Geometry check sheet. Reference: drawing and pictorial views, mm from the part's lowest x, y, z. Coordinates: 2 decimals unless noted, no trailing zeros. Write each loop counter-clockwise with the first axis right and the second up, starting at its lowest first coordinate (ties: lowest second). Pieces come first, ordered by that corner, then holes. Notation, with made-up numbers: (16.25, 57) -> (39.25, 57) arc R15 ccw to (39.25, 69) -> close; hole circle Ø4 at (-21.5, 45). An arc over 180 degrees is marked (long way). Use a Markdown table: item, result.
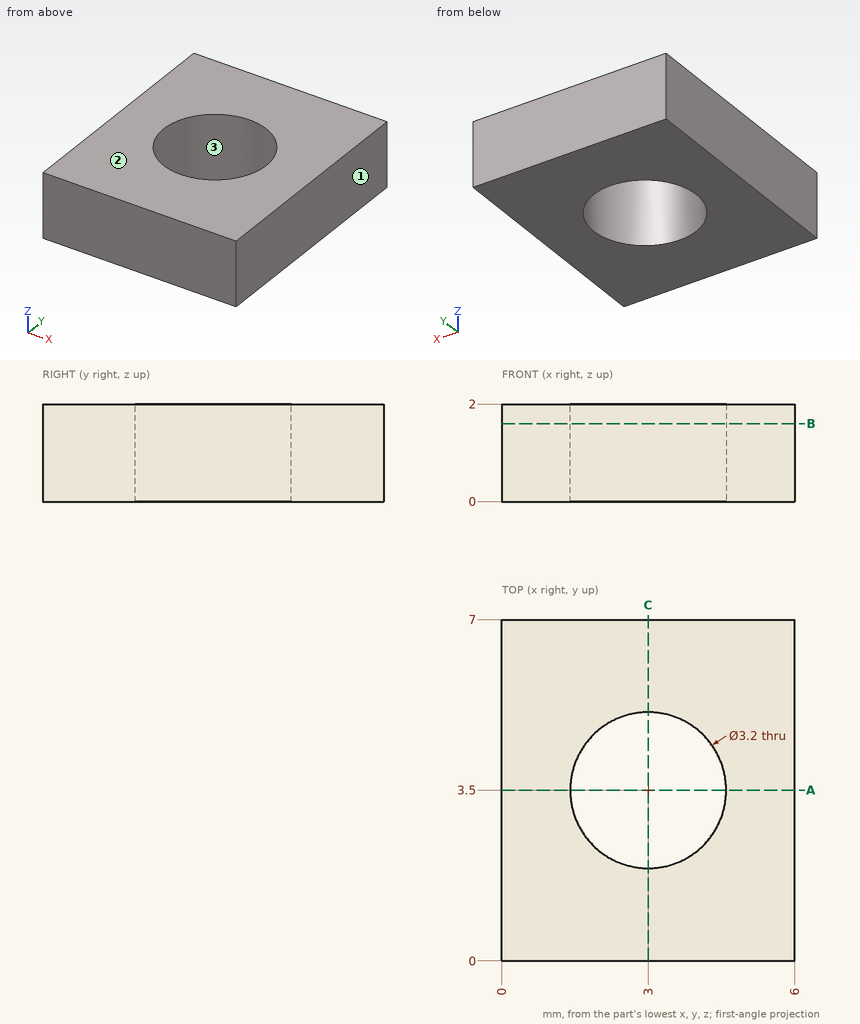
Item 1: Section check B-B on z = 1.6. Record the boundary of the cut face in (x, y), then the cut area to 3 significant figures.
Answer block:
| item | result |
|---|---|
| outline | (0, 0) -> (6, 0) -> (6, 7) -> (0, 7) -> close; hole circle Ø3.2 at (3, 3.5) |
| area | 34.0 mm^2 |
Item 2: Section check C-C on x = 3. Record the boundary of the cut face in (y, z), then the cut area to 3 significant figures.
Answer block:
| item | result |
|---|---|
| outline | (0, 0) -> (1.9, 0) -> (1.9, 2) -> (0, 2) -> close; (5.1, 0) -> (7, 0) -> (7, 2) -> (5.1, 2) -> close |
| area | 7.60 mm^2 |
Item 3: Section check A-A on y = 3.5. Record the boundary of the cut face in (x, z), then the cut area to 3 significant figures.
Answer block:
| item | result |
|---|---|
| outline | (0, 0) -> (1.4, 0) -> (1.4, 2) -> (0, 2) -> close; (4.6, 0) -> (6, 0) -> (6, 2) -> (4.6, 2) -> close |
| area | 5.60 mm^2 |
Item 4: Thickness scan on L1, parallel to Y at x = 3, z = 1.5; L2, parallel to Y at x = 4.45, z = 1.65; L3, parallel to X at y = 2.5, z = 0.2. Record the ranges inside material, lowest first. Write a range as [from, to].
Answer block:
| item | result |
|---|---|
| L1 | y = [0, 1.9], [5.1, 7] |
| L2 | y = [0, 2.82], [4.18, 7] |
| L3 | x = [0, 1.75], [4.25, 6] |
Item 5: Mould release check, pull along X, two halves, no side actions. Record for the marked faces 1, 2 and 3: +X half, -X half, draft (parallel to the pull), parting line (faces both ways), or undercut.
Answer block:
| item | result |
|---|---|
| face 1 | +X half |
| face 2 | draft |
| face 3 | undercut |
